```python
from build123d import *

# Parameters (mm, degrees)
SKETCH1_R           = 5
BOSS_EXTRUDE1_DEPTH = 22
CUT_EXTRUDE1_START  = -6
CUT_EXTRUDE1_DEPTH  = 6
SKETCH3_R           = 3
BOSS_EXTRUDE2_DEPTH = 20
SKETCH4_R           = 10
BOSS_EXTRUDE3_DEPTH = 6
SKETCH5_R           = 22.5
BOSS_EXTRUDE4_DEPTH = 3
SKETCH6_R           = 2
CUT_EXTRUDE2_DEPTH  = 3


with BuildPart() as part:
    # Sketch1 → Boss-Extrude1 (new body)
    with BuildSketch(Plane.XY):
        Circle(SKETCH1_R)
    extrude(amount=BOSS_EXTRUDE1_DEPTH)

    # Sketch2 → Cut-Extrude1 (cut)
    with BuildSketch(Plane.XY.offset(22).offset(CUT_EXTRUDE1_START)):
        with BuildLine():
            Line((2.638277831, 4.247292089), (-4.299208102, 2.552804281))
            ThreePointArc((-4.299208102, 2.552804281), (-1.186378765, 4.857211693), (2.638277831, 4.247292089))
        make_face()
        with BuildLine():
            Line((-2.638277831, -4.247292089), (4.299208102, -2.552804281))
            ThreePointArc((4.299208102, -2.552804281), (1.186378765, -4.857211693), (-2.638277831, -4.247292089))
        make_face()
    extrude(amount=CUT_EXTRUDE1_DEPTH, mode=Mode.SUBTRACT)

    # Sketch3 → Boss-Extrude2 (add)
    with BuildSketch(Plane.XY.offset(22)):
        Circle(SKETCH3_R)
    extrude(amount=BOSS_EXTRUDE2_DEPTH)

    # Sketch4 → Boss-Extrude3 (add)
    with BuildSketch(Plane(origin=(0, 0, 0), x_dir=(-1, 0, 0), z_dir=(0, 0, -1))):
        Circle(SKETCH4_R)
    extrude(amount=BOSS_EXTRUDE3_DEPTH)

    # Sketch5 → Boss-Extrude4 (add)
    with BuildSketch(Plane(origin=(0, 0, -6), x_dir=(-1, 0, 0), z_dir=(0, 0, -1))):
        Circle(SKETCH5_R)
    extrude(amount=BOSS_EXTRUDE4_DEPTH)

    # Sketch6 → Cut-Extrude2 (cut)
    with BuildSketch(Plane(origin=(0, 0, -9), x_dir=(-1, 0, 0), z_dir=(0, 0, -1))):
        with Locations((-16, 0)):
            Circle(SKETCH6_R)
        with Locations((0, 16)):
            Circle(SKETCH6_R)
        with Locations((16, 0)):
            Circle(SKETCH6_R)
        with Locations((0, -16)):
            Circle(SKETCH6_R)
    extrude(amount=-CUT_EXTRUDE2_DEPTH, mode=Mode.SUBTRACT)


solid = part.part
```
Here's how the part is built. I have some questions about the finished solid (model axes, mm). A direction names the side the tool comes from. Give positions to 0.01 mm unless a question says otherwise; leave off trailing zeros. Write each loop counter-clockwise with the first axis right and the second up, starting at its lowest first coordinate (ties: lowest second). Pieces come first, ordered by that corner, then holes. Notation, with made-up numbers: M 35.25,42 L 64.25,42 A17 cw 64.25,58 Z; hole C -5,-1 d10. An arc over 180 degrees is marked long. Put each result on its own line as item: value. Start each with the question number.
Item 1: If we section it at D-D, the plane x = 0: Write out the boundary of the cut face in (y, z).
Item 2: If we section it at B-B, the plane x = 16: Write out the boundary of the cut face in (y, z).
Item 3: On a 3-axis mill with a long thin cutter (end or side, diameter ignored), from which of +Z, -Z, +X, -X, +Y, -Y can I reach the whole of each face in a straight line? I mean faces 1 (the cylindrical face through (-3, 0, 32)), 2 (the cylindrical face through (-14.4, -1.2, -7.5)), 3 (the flat face through (-0.782, 3.412, 18.958)), 4 (the flat face through (1, -4, 16)), 5 (the flat face through (0, 0, 42)). Say none if no direction works.
Item 4: If we section it at A-A, the plane y = 0: Write out the boundary of the cut face in (x, z).
Item 5: Thinking about a two-plate mould opening in X: for faces 6 (the cylindrical face through (17.6, -1.2, -7.5)), 7 (the flat face through (0.782, -3.412, 18.958)), 8 (the flat face through (0, 0, -9)), which applies, +X half, -X half, draft (parallel to the pull), parting line (faces both ways), or undercut?
Item 6: I need wall thicknesses on L1, parallel to Y at x = 0, z = -7; L2, parallel to Z at x = -12, y = -1; L3, parallel to Z at x = -4, y = 8. Which ranges of each line are inside material? Lowest first, please. Write a range as from..to.
Item 7: Will these pins go through, and if not, where does the flat tip stop? pin 1 (1 mm diameter, centred on y = 2, z = 15, fed in from +X); pin 2 (10 mm diameter, centred on x = -1, z = 16.5, fed in from +Y); pin 3 (6 mm diameter, centred on x = -7.5, y = 3, fed in from +Z); pin 4 (12 mm diameter, centred on y = 12, z = 29, fed in from +X) (3 decimals).
Values:
1. outline: M -22.5,-9 L -18,-9 L -18,-6 L -22.5,-6 Z; M -14,-9 L 14,-9 L 14,-6 L 10,-6 L 10,0 L 5,0 L 5,16 L 3.6,16 L 3.6,22 L 3,22 L 3,42 L -3,42 L -3,22 L -3.6,22 L -3.6,16 L -5,16 L -5,0 L -10,0 L -10,-6 L -14,-6 Z; M 18,-9 L 22.5,-9 L 22.5,-6 L 18,-6 Z
2. outline: M -15.82,-9 L -2,-9 L -2,-6 L -15.82,-6 Z; M 2,-9 L 15.82,-9 L 15.82,-6 L 2,-6 Z
3. face 1: +Z
3. face 2: +Z, -Z
3. face 3: +Z, -X, +Y
3. face 4: +Z, +X, -Y
3. face 5: +Z, +X, -X, +Y, -Y
4. outline: M -22.5,-9 L -18,-9 L -18,-6 L -22.5,-6 Z; M -14,-9 L 14,-9 L 14,-6 L 10,-6 L 10,0 L 5,0 L 5,22 L 3,22 L 3,42 L -3,42 L -3,22 L -5,22 L -5,0 L -10,0 L -10,-6 L -14,-6 Z; M 18,-9 L 22.5,-9 L 22.5,-6 L 18,-6 Z
5. face 6: undercut
5. face 7: +X half
5. face 8: draft
6. L1: -22.5..-18, -14..14, 18..22.5
6. L2: -9..-6
6. L3: -9..0
7. pin 1: x = 4.77
7. pin 2: y = 5
7. pin 3: z = 0
7. pin 4: through
